```python
from build123d import *

# Parameters (mm, degrees)
SKETCH1_R                 = 4
BOSS_EXTRUDE1_DEPTH       = 3
SKETCH1_3_R               = 4
BOSS_EXTRUDE2_DEPTH       = 340
BOSS_EXTRUDE3_START       = -30
BOSS_EXTRUDE3_OUTLINE_W   = 34
BOSS_EXTRUDE3_OUTLINE_H   = 30
BOSS_EXTRUDE3_OUTLINE_R   = 4
BOSS_EXTRUDE3_OUTLINE_W_2 = 30
BOSS_EXTRUDE3_OUTLINE_H_2 = 30.979171587
BOSS_EXTRUDE3_DEPTH       = 30
SKETCH5_W                 = 100
SKETCH5_H                 = 366
BOSS_EXTRUDE4_DEPTH       = 3
SKETCH6_W                 = 102
SKETCH6_H                 = 116
BOSS_EXTRUDE6_DEPTH       = 3


# Read off the part's stored shape, not the designer's step: Boss-Extrude3
with BuildPart() as part:
    # Sketch1 → Boss-Extrude1 (new body)
    with BuildSketch(Plane(origin=(0, 0, 0), x_dir=(1, 0, 0), z_dir=(0, 1, 0))):
        with BuildLine():
            Line((0, 84), (0, 0))
            Line((0, 0), (168.5, 0))
            Line((168.5, 0), (168.5, 84.179067966))
            Line((168.5, 84.179067966), (104.941145125, 84.111522833))
            ThreePointArc((104.941145125, 84.111522833), (80.098432068, 106.08513446), (55.302478571, 84.058770934))
            Line((55.302478571, 84.058770934), (0, 84))
        make_face()
        with Locations(Location((80.125, 42.085148577, 0), (0, 0, 270))):
            Circle(SKETCH1_R, mode=Mode.SUBTRACT)
        with Locations(Location((80.125, 81.085148577, 0), (0, 0, 270))):
            Circle(SKETCH1_R, mode=Mode.SUBTRACT)
    extrude(amount=BOSS_EXTRUDE1_DEPTH)

    # Sketch1<3> → Boss-Extrude2 (add)
    with BuildSketch(Plane(origin=(0, 0, 0), x_dir=(1, 0, 0), z_dir=(0, 1, 0))):
        with BuildLine():
            ThreePointArc((82.767561665, 84.087958569), (80.120749131, 85.085146319), (77.476062031, 84.082335198))
            Line((77.476062031, 84.082335198), (82.767561665, 84.087958569))
        make_face()
        with BuildLine():
            Line((82.767561665, 84.087958569), (77.476062031, 84.082335198))
            ThreePointArc((77.476062031, 84.082335198), (78.481186123, 77.438523297), (84.125, 81.085148577))
            ThreePointArc((84.125, 81.085148577), (83.769876312, 82.732836858), (82.767561665, 84.087958569))
        make_face()
        with Locations(Location((80.125, 42.085148577, 0), (0, 0, 270))):
            Circle(SKETCH1_3_R)
    extrude(amount=BOSS_EXTRUDE2_DEPTH)

    # Boss-Extrude3 outline → Boss-Extrude3 (add)
    # profile 1 of 2: a face of its own
    with BuildSketch(Plane.XY.offset(-27).offset(BOSS_EXTRUDE3_START)):
        with Locations((28.275525376, -15)):
            Rectangle(BOSS_EXTRUDE3_OUTLINE_W, BOSS_EXTRUDE3_OUTLINE_H)
        with Locations((28.275525376, -15)):
            Circle(BOSS_EXTRUDE3_OUTLINE_R, mode=Mode.SUBTRACT)
    # profile 2 of 2: a face of its own
    with BuildSketch(Plane.XY.offset(-27).offset(BOSS_EXTRUDE3_START)):
        with Locations((140.075525376, -15.489585794)):
            Rectangle(BOSS_EXTRUDE3_OUTLINE_W_2, BOSS_EXTRUDE3_OUTLINE_H_2)
        with Locations((140.075525376, -21)):
            Circle(BOSS_EXTRUDE3_OUTLINE_R, mode=Mode.SUBTRACT)
    extrude(amount=BOSS_EXTRUDE3_DEPTH)

    # Sketch5 → Boss-Extrude4 (add)
    with BuildSketch(Plane(origin=(168.5, 0, 0), x_dir=(0, 0, -1), z_dir=(1, 0, 0))):
        with Locations((42.089533983, 173)):
            Rectangle(SKETCH5_W, SKETCH5_H)
    extrude(amount=BOSS_EXTRUDE4_DEPTH)

    # Sketch6 → Boss-Extrude6 (add)
    with BuildSketch(Plane(origin=(0, 340, 0), x_dir=(1, 0, 0), z_dir=(0, 1, 0))):
        with Locations((117.5, 42.085148577)):
            Rectangle(SKETCH6_W, SKETCH6_H)
    extrude(amount=BOSS_EXTRUDE6_DEPTH)


solid = part.part
```
Here's how the part is built. I have some questions about the finished solid (model axes, mm). A direction names the side the tool comes from. Round coordinates to 2 decimals unless told otherwise and drop trailing zeros. Order: outer loops, then holes, each group sorted by start corner. A loop starts at its lowest first (then second) coordinate and runs counter-clockwise, first axis right, second up. Notation, with made-up numbers: M 79,58.5 L 109,58.5 A25 cw 109,88.5 Z; hole C 34,88.25 d3. An arc over 180 degrees is marked long. Answer in a Markdown table with one row per item.
Item 1: For faces 1 (the face through (11.276, -15, -42)), 2 (the face through (80.61, 1.48, -106.08)), 3 (the face through (140, -15, -57)), which set-ups out of +Z, -Z, +X, -X, +Y, -Y let a thin tool reach every point of the face, with its end or its side?
A:
| item | result |
|---|---|
| face 1 | +Z, -Z, -X, -Y |
| face 2 | -Z, -Y |
| face 3 | -Z, -X, -Y |
Item 2: Imagine slicing it at B-B, the plane x = 101. Write out the boundary of the cut face in (y, z), and give its area (3 significant figures).
A:
| item | result |
|---|---|
| outline | M 0,-94.84 L 3,-94.84 L 3,0 L 0,0 Z; M 340,-100.09 L 343,-100.09 L 343,15.91 L 340,15.91 Z |
| area | 633 mm2 |
Item 3: Thinking about a two-plate mould opening in Y: for faces 4 (the face through (171.5, 176, -41)), 5 (the face through (28, -30, -42)), 6 (the face through (117, 343, -43)), 7 (the face through (32.09, -13.8, -42.21)), which applies, +Y half, -Y half, draft (parallel to the pull), parting line (faces both ways), or undercut?
A:
| item | result |
|---|---|
| face 4 | draft |
| face 5 | -Y half |
| face 6 | +Y half |
| face 7 | undercut |
Item 4: Imagine slicing it at C-C, the plane y = 184. Write out the boundary of the cut face in (x, z) (3 decimals), and give its area (3 significant figures).
A:
| item | result |
|---|---|
| outline | C 80.125,-81.085 d8; C 80.125,-42.085 d8; M 168.5,-92.09 L 171.5,-92.09 L 171.5,7.91 L 168.5,7.91 Z |
| area | 401 mm2 |
Item 5: Imagine slicing it at A-A, the plane z = -34. Write out the boundary of the cut face in (x, y), and give its area (3 significant figures).
A:
| item | result |
|---|---|
| outline | M 0,0 L 11.28,0 L 11.28,-30 L 45.28,-30 L 45.28,0 L 125.08,0 L 125.08,-30.98 L 155.08,-30.98 L 155.08,0 L 168.5,0 L 168.5,-10 L 171.5,-10 L 171.5,356 L 168.5,356 L 168.5,343 L 66.5,343 L 66.5,340 L 168.5,340 L 168.5,3 L 0,3 Z; hole C 28.28,-15 d8; hole C 140.08,-21 d8 |
| area | 3,760 mm2 |
Item 6: If I drill on L1, parallel to Y at x = 109, z = -83.5; L2, parallel to Y at x = 63, z = -3; L3, parallel to Y at x = 141, z = -27.5, over which ranges is the centre line in solid material (lowest first)? Write a range as from..to.
A:
| item | result |
|---|---|
| L1 | y = 0..3, 340..343 |
| L2 | y = 0..3 |
| L3 | y = -30.98..-24.89, -17.11..3, 340..343 |
Item 7: I'm going to push flat-ended pins straight in: pin 1 (15 mm diameter, centred on y = -8.5, z = -47.5, fed in from -X); pin 2 (0.9 mm diameter, centred on y = 342, z = 10.5, fed in from +X); pin 3 (2.5 mm diameter, centred on x = 170.5, z = -48, fed in from -Y). Where does each tip first touch, or does it pass through?
A:
| item | result |
|---|---|
| pin 1 | stops at x = 11.28 |
| pin 2 | stops at x = 168.5 |
| pin 3 | stops at y = -10 |
Item 8: Imagine slicing it at D-D, the plane z = -66. Write out the boundary of the cut face in (x, y).
A:
| item | result |
|---|---|
| outline | M 0,0 L 168.5,0 L 168.5,-10 L 171.5,-10 L 171.5,356 L 168.5,356 L 168.5,343 L 66.5,343 L 66.5,340 L 168.5,340 L 168.5,3 L 0,3 Z |
